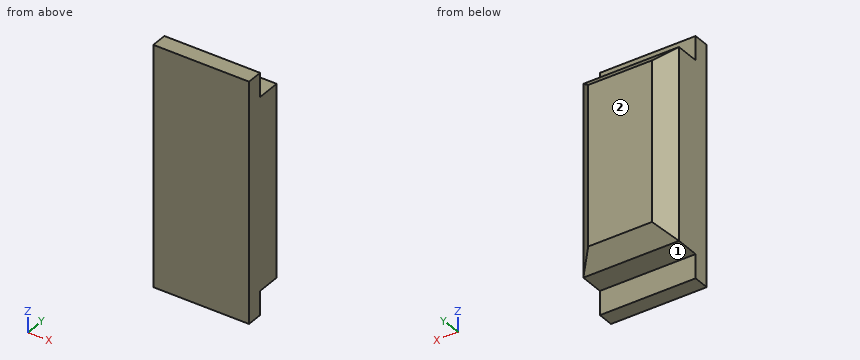
from build123d import *

# Parameters (mm, degrees)
SKETCH1_W           = 12
SKETCH1_H           = 30
BOSS_EXTRUDE1_DEPTH = 2
SKETCH2_W           = 12
SKETCH2_H           = 24
BOSS_EXTRUDE2_DEPTH = 5
CHAMFER1_SIZE       = 2


with BuildPart() as part:
    # Sketch1 → Boss-Extrude1 (new body)
    with BuildSketch(Plane(origin=(0, 0, 0), x_dir=(1, 0, 0), z_dir=(0, 1, 0))):
        with Locations((6, 15)):
            Rectangle(SKETCH1_W, SKETCH1_H)
    extrude(amount=BOSS_EXTRUDE1_DEPTH)

    # Sketch2 → Boss-Extrude2 (add)
    with BuildSketch(Plane(origin=(0, 2, 0), x_dir=(1, 0, 0), z_dir=(0, 1, 0))):
        with Locations((6, 15)):
            Rectangle(SKETCH2_W, SKETCH2_H)
    extrude(amount=BOSS_EXTRUDE2_DEPTH)

    # Chamfer1
    chamfer1_edges = [part.edges().sort_by_distance(p)[0] for p in [
        (0, 7, -15),
        (6, 7, -3),
        (12, 7, -15),
        (6, 7, -27),
    ]]
    chamfer(chamfer1_edges, length=CHAMFER1_SIZE)


solid = part.part
Geometry check sheet. Reference: the model listing, model coordinates, mm. Face numbers are marked on the shaded views. A direction names the side the tool comes from. Round coordinates to 2 decimals unless told otherwise and drop trailing zeros. Write each loop counter-clockwise with the first axis right and the second up, starting at its lowest first coordinate (ties: lowest second). Pieces come first, ordered by that corner, then holes. Notation, with made-up numbers: (18.5, 86.25) -> (48.5, 86.25) arc R8 ccw to (48.5, 95.25) -> close; hole circle Ø4 at (63.25, 20). An arc over 180 degrees is marked (long way). One line per item, written item: value. Start each with the question number.
(1) Cross-section at C-C, the plane y = 6. Record the cut outline in (x, z), and give its area (3 significant figures).
(2) Cross-section at A-A, the plane z = -23.75. Record the cut outline in (x, y), and give its area (3 significant figures).
(3) Go/stop test with flat-tipped pins: pin 1 Ø4 at (x, y) = (5.5, 6) entering from -Z; pin 2 Ø2.5 at (x, z) = (3.5, -1.5) entering from +Y; pin 3 Ø0.9 at (x, y) = (4.5, 4) entering from +Z. Record where each tip stops, or that it passes through.
(4) Cross-section at B-B, the plane x = 10.5. Record the cut outline in (y, z).
(5) Access from +Z, -Z, +X, -X, +Y, -Y to the whole of each face (thin tool, end or side, straight path). Record for the marked faces 1 and 2.
(6) Cross-section at D-D, the plane z = -3.5. Record the cut outline in (x, y).
(7) Scan lines: line 1 (Z direction, x = 7.25, y = 2.25); line 2 (Y direction, x = 8, z = -1.25); line 3 (Y direction, x = 6.5, z = -3.75). Record each from-to range of solid material in increasing order. Write a range as [from, to].
Answer:
1. outline: (1, -26) -> (11, -26) -> (11, -4) -> (1, -4) -> close
1. area: 220 mm²
2. outline: (0, 0) -> (12, 0) -> (12, 5) -> (10, 7) -> (2, 7) -> (0, 5) -> close
2. area: 80.0 mm²
3. pin 1: z = -27
3. pin 2: y = 2
3. pin 3: z = -3
4. outline: (0, -30) -> (2, -30) -> (2, -27) -> (5, -27) -> (6.5, -25.5) -> (6.5, -4.5) -> (5, -3) -> (2, -3) -> (2, 0) -> (0, 0) -> close
5. face 1: -Z, +X, -X, +Y
5. face 2: +Z, -Z, +X, -X, +Y
6. outline: (0, 0) -> (12, 0) -> (12, 5) -> (11.5, 5.5) -> (0.5, 5.5) -> (0, 5) -> close
7. line 1: [-27, -3]
7. line 2: [0, 2]
7. line 3: [0, 5.75]
